Design review of the part built by this model. Coordinates are the model's own, in mm. Face numbers are marked on the shaded views. Coordinates: 2 decimals unless noted, no trailing zeros. Write each loop counter-clockwise with the first axis right and the second up, starting at its lowest first coordinate (ties: lowest second). Pieces come first, ordered by that corner, then holes. Notation, with made-up numbers: (24, 14) - (30, 14) arc R24 cw to (30, 46) - close; hole circle Ø11 at (45, 80.25). An arc over 180 degrees is marked (long way). Use a Markdown table: item, result.
from build123d import *

# Parameters (mm, degrees)
SKETCH1_R           = 12.5
SKETCH1_R_2         = 3
BOSS_EXTRUDE1_DEPTH = 12
SKETCH2_R           = 3
BOSS_EXTRUDE2_DEPTH = 1
CHAMFER1_SIZE       = 6
CHAMFER1_SIZE2      = 8.56888804


with BuildPart() as part:
    # Sketch1 → Boss-Extrude1 (new body)
    with BuildSketch(Plane.XY):
        Circle(SKETCH1_R)
        Circle(SKETCH1_R_2, mode=Mode.SUBTRACT)
    extrude(amount=BOSS_EXTRUDE1_DEPTH)

    # Sketch2 → Boss-Extrude2 (add)
    with BuildSketch(Plane.XY.offset(12)):
        Circle(SKETCH2_R)
    extrude(amount=-BOSS_EXTRUDE2_DEPTH)

    # Chamfer1
    chamfer1_edges = [part.edges().sort_by_distance(p)[0] for p in [
        (-12.5, 0, 0),
    ]]
    chamfer1_side = [part.faces().sort_by_distance(p)[0] for p in [
        (-12.146446609, 0, 0),
    ]]
    chamfer(chamfer1_edges, length=CHAMFER1_SIZE, length2=CHAMFER1_SIZE2, reference=chamfer1_side[0])


solid = part.part
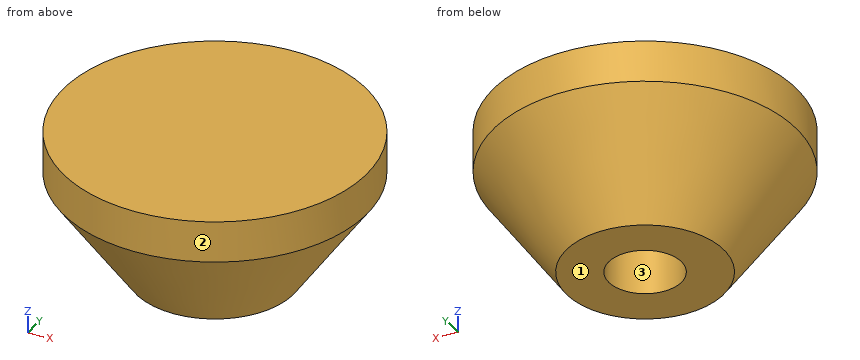
(1) Take a section at C-C on z = 8. Write out the cut boundary in (x, y), and give its area (3 significant figures).
Determined:
| item | result |
|---|---|
| outline | circle Ø24.2 at (0, 0); hole circle Ø6 at (0, 0) |
| area | 432 mm2 |
(2) For pin 1 (3 mm diameter, centred on x = -7.5, z = 5.5, fed in from +Y); pin 2 (4 mm diameter, centred on y = 3, z = 3, fed in from +X); pin 3 (3 mm diameter, centred on x = 0, y = 1, fed in from -Z), all flat-tipped, find the tip position at first contact; note any pin that passes through.
Determined:
| item | result |
|---|---|
| pin 1 | y = 9.04 |
| pin 2 | x = 9.64 |
| pin 3 | z = 11 |
(3) For L1, parallel to Y at x = 0, z = 8; L2, parallel to Y at x = -1.25, z = 4.75; L3, parallel to Z at x = 0.25, y = -0.25, list the stretches that pass through material, from the lowest coordinate up. Write a range as from..to.
Determined:
| item | result |
|---|---|
| L1 | -12.1..-3, 3..12.1 |
| L2 | -9.75..-2.73, 2.73..9.75 |
| L3 | 11..12 |
(4) Draft analysis for pull direction X (two halves, no side actions). For the marked faces 1, 2 and 3, state which applies: +X half, -X half, draft (parallel to the pull), parting line (faces both ways), or undercut.
Determined:
| item | result |
|---|---|
| face 1 | draft |
| face 2 | parting line |
| face 3 | undercut |
(5) Take a section at A-A on y = 0. Write out the cut boundary in (x, z).
Determined:
| item | result |
|---|---|
| outline | (-12.5, 8.57) - (-6.5, 0) - (-3, 0) - (-3, 11) - (3, 11) - (3, 0) - (6.5, 0) - (12.5, 8.57) - (12.5, 12) - (-12.5, 12) - close |
